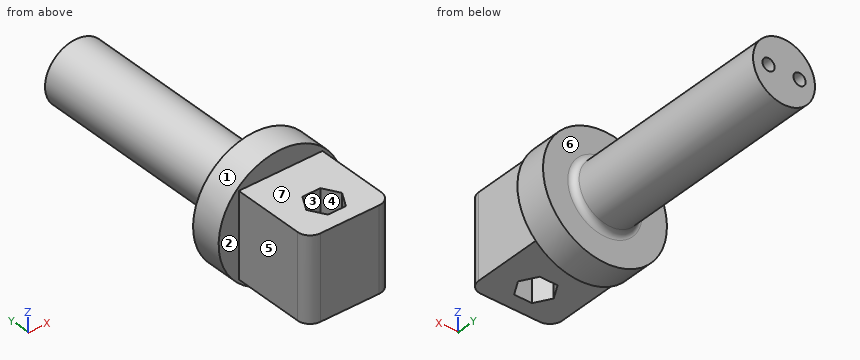
from build123d import *

# Parameters (mm, degrees)
BOSS_EXTRUDE1_DEPTH       = 34.31697226
SKETCH4_R                 = 25.4
BOSS_EXTRUDE2_DEPTH       = 12.7
SKETCH6_R                 = 12.7
BOSS_EXTRUDE3_DEPTH       = 88.9
CUT_EXTRUDE1_DEPTH        = 145.667412963
FILLET1_R                 = 5.08
FILLET2_R                 = 2.54
M6X1_0_TAPPED_HOLE1_D     = 5
M6X1_0_TAPPED_HOLE1_DEPTH = 38.1
M6X1_0_TAPPED_HOLE1_TIP   = 1.502151548


with BuildPart() as part:
    # Sketch3 → Boss-Extrude1 (new body)
    with BuildSketch(Plane(origin=(0, 0, 0), x_dir=(1, 0, 0), z_dir=(0, 1, 0))):
        Polygon((17.145, 0), (17.145, 17.145), (0, 17.145), (-17.145, 17.145), (-17.145, 0), (-17.145, -17.145), (0, -17.145), (17.145, -17.145), align=None)
    extrude(amount=BOSS_EXTRUDE1_DEPTH)

    # Sketch4 → Boss-Extrude2 (add)
    with BuildSketch(Plane(origin=(0, 34.31697226, 0), x_dir=(1, 0, 0), z_dir=(0, 1, 0))):
        with Locations(Location((0, 0, 0), (0, 0, 270))):
            Circle(SKETCH4_R)
    extrude(amount=BOSS_EXTRUDE2_DEPTH)

    # Sketch6 → Boss-Extrude3 (add)
    with BuildSketch(Plane(origin=(0, 47.01697226, 0), x_dir=(1, 0, 0), z_dir=(0, 1, 0))):
        with Locations(Location((0, 0, 0), (0, 0, 270))):
            Circle(SKETCH6_R)
    extrude(amount=BOSS_EXTRUDE3_DEPTH)

    # Sketch7 → Cut-Extrude1 (cut, through all)
    with BuildSketch(Plane.XY.offset(17.145)):
        Polygon((7.332348419, 12.7), (3.666174209, 19.05), (-3.666174209, 19.05), (-7.332348419, 12.7), (-3.666174209, 6.35), (3.666174209, 6.35), align=None)
    extrude(amount=-CUT_EXTRUDE1_DEPTH, mode=Mode.SUBTRACT)

    # Fillet1
    fillet1_edges = [part.edges().sort_by_distance(p)[0] for p in [
        (17.145, 0, 0),
        (-17.145, 0, 0),
    ]]
    fillet(fillet1_edges, radius=FILLET1_R)

    # Fillet2
    fillet2_edges = [part.edges().sort_by_distance(p)[0] for p in [
        (0, 47.01697226, -12.7),
    ]]
    fillet(fillet2_edges, radius=FILLET2_R)

    # M6x1.0 Tapped Hole1
    with Locations(Plane(origin=(0, 135.91697226, 0), x_dir=(1, 0, 0), z_dir=(0, 1, 0))):
        with Locations((6.35, 0), (-6.35, 0)):
            Hole(M6X1_0_TAPPED_HOLE1_D / 2, depth=M6X1_0_TAPPED_HOLE1_DEPTH)
            with Locations((0, 0, -(M6X1_0_TAPPED_HOLE1_DEPTH + M6X1_0_TAPPED_HOLE1_TIP / 2))):  # 118° drill point
                Cone(0, M6X1_0_TAPPED_HOLE1_D / 2, M6X1_0_TAPPED_HOLE1_TIP, mode=Mode.SUBTRACT)


solid = part.part
Here's how the part is built. I have some questions about the finished solid (model axes, mm). Face numbers are marked on the shaded views. A direction names the side the tool comes from. Coordinates: 2 decimals unless noted, no trailing zeros. Loops run counter-clockwise (first coordinate to the right, second up) from the corner with the lowest first, then second, coordinate; pieces in that order, holes last. Notation, with made-up numbers: (-3, 23.25) -> (17, 23.25) arc R13 ccw to (17, 47.25) -> close; hole circle Ø9 at (-11, 56.25). An arc over 180 degrees is marked (long way). Use one line per item in the form item = value. Start each with the question number.
(1) Will these pins go through, and if not, where does the flat tip stop? pin 1 (8 mm diameter, centred on x = 12.5, y = 80, fed in from +Z); pin 2 (1.5 mm diameter, centred on y = 121.5, z = 0, fed in from +X); pin 3 (14.5 mm diameter, centred on y = 26.5, z = -3.5, fed in from -X) (3 decimals); pin 4 (8 mm diameter, centred on x = 6.35, z = 0, fed in from +Y).
(2) Please list where these lines run through material, in increasing order: line 1 along Y through (x, z) = (-8.5, -17); line 2 along Z through (x, y) = (2, 32) (3 decimals); line 3 along Y through (x, z) = (4, -4.5).
(3) If we section it at B-B (y = 113): Please give me the cut outline in (x, z).
(4) On a 3-axis mill with a long thin cutter (end or side, diameter ignored), from which of +Z, -Z, +X, -X, +Y, -Y can I reach the whole of each face in a straight line? I mean the marked faces 4, 5, 6 and 7. Say none if no direction works.
(5) If we section it at C-C (x = -20): Please give me the cut outline in (y, z), then the cut area to 3 significant figures.
(6) If we section it at A-A (y = 17): Please give me the cut outline in (x, z) (3 decimals), then the cut area to 3 significant figures.
(7) If we section it at D-D (y = 86.5): Please give me the cut outline in (x, z), then the cut area to 3 significant figures.
(8) We'd pull the mould along X, two halves only. Please class the marked faces 1, 2 and 3: pulls with the +X half, pulls with the -X half, needs draft (parallel to the pull), parting line crosses it, or undercut.
Verdict:
q1.pin_1 = 9.44
q1.pin_2 = 12.7
q1.pin_3 = -17.145
q1.pin_4 = 135.92
q2.line_1 = 0 to 47.02
q2.line_2 = -17.145 to 17.145
q2.line_3 = 0 to 6.93, 18.47 to 135.92
q3.outline = circle Ø25.4 at (0, 0); hole circle Ø5 at (-6.35, 0); hole circle Ø5 at (6.35, 0)
q4.face_4 = +Z, -Z
q4.face_5 = +Z, -Z, -X, -Y
q4.face_6 = +Y
q4.face_7 = +Z, +X, -X, -Y
q5.outline = (34.32, -15.66) -> (47.02, -15.66) -> (47.02, 15.66) -> (34.32, 15.66) -> close
q5.area = 398 mm²
q6.outline = (-17.145, -17.145) -> (-4.85, -17.145) -> (-4.85, 17.145) -> (-17.145, 17.145) -> close; (4.85, -17.145) -> (17.145, -17.145) -> (17.145, 17.145) -> (4.85, 17.145) -> close
q6.area = 843 mm²
q7.outline = circle Ø25.4 at (0, 0)
q7.area = 507 mm²
q8.face_1 = parting line crosses it
q8.face_2 = needs draft
q8.face_3 = undercut
